Verification items for this drawing (mm, ordinates from the low corner). A direction names the side the tool comes from. Give positions to 0.01 mm unless a question says otherwise; leave off trailing zeros. Order: outer loops, then holes, each group sorted by start corner. A loop starts at its lowest first (then second) coordinate and runs counter-clockwise, first axis right, second up. Notation, with made-up numbers: (-7.5, -18) -> (7.5, -18) arc R19 ccw to (7.5, 19) -> close; hole circle Ø11 at (11.25, 9). An arc over 180 degrees is marked (long way). One line per question, with ' | ' between items.
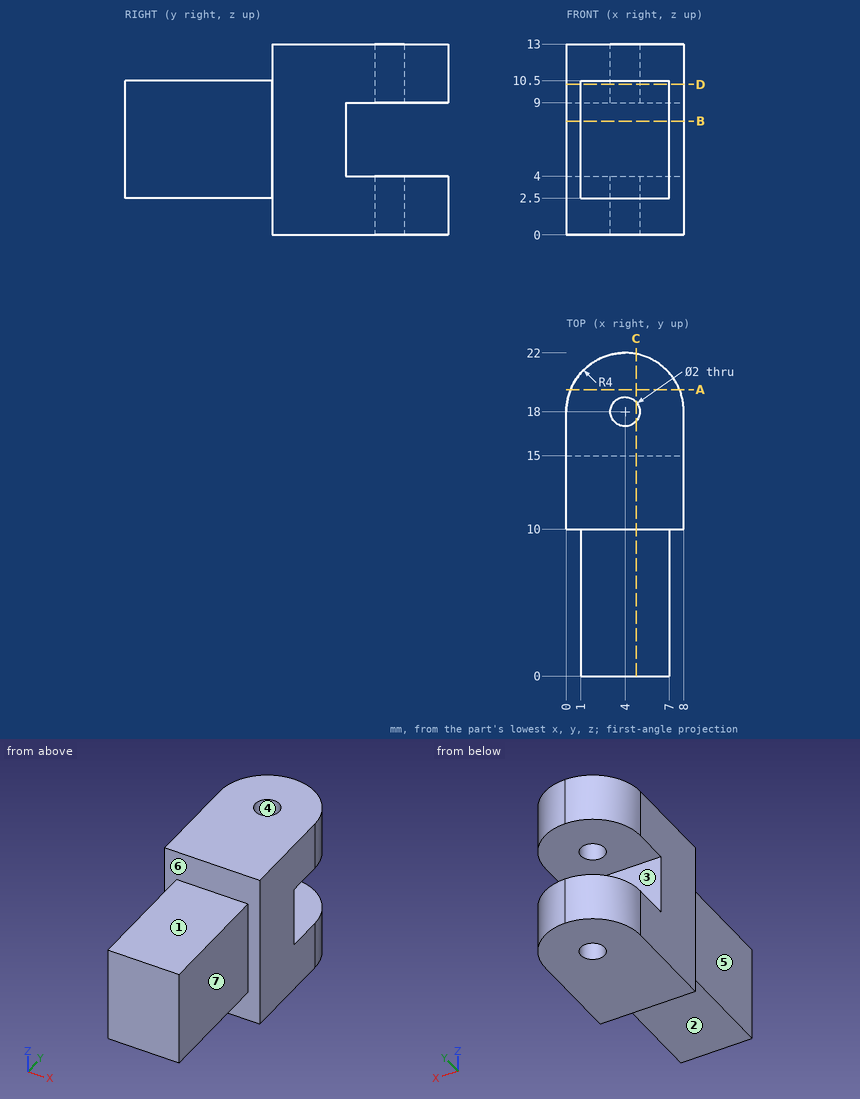
Q1. Section check B-B (z = 7.75). Enter the section's corners in (x, y), and give its area (3 significant figures).
Result sheet:
outline: (0, 10) -> (1, 10) -> (1, 0) -> (7, 0) -> (7, 10) -> (8, 10) -> (8, 15) -> (0, 15) -> close | area: 100 mm2
Q2. Access from +Z, -Z, +X, -X, +Y, -Y to the whole of each face (thin tool, end or side, straight path). Record for the marked faces 1, 2 and 3.
Result sheet:
face 1: +Z, +X, -X, -Y | face 2: -Z, +X, -X, -Y | face 3: +X, -X, +Y
Q3. Mould release check, pull along X, two halves, no side actions. Record for the marked faces 4, 5, 6 and 7: pulls with the +X half, pulls with the -X half, needs draft (parallel to the pull), parting line crosses it, or undercut.
Result sheet:
face 4: undercut | face 5: pulls with the -X half | face 6: needs draft | face 7: pulls with the +X half
Q4. Section check A-A (y = 19.5). Enter the section's corners in (x, z).
Result sheet:
outline: (0.29, 0) -> (7.71, 0) -> (7.71, 4) -> (0.29, 4) -> close; (0.29, 9) -> (7.71, 9) -> (7.71, 13) -> (0.29, 13) -> close
Q5. Section check D-D (z = 10.25). Enter the section's corners in (x, y).
Result sheet:
outline: (0, 10) -> (1, 10) -> (1, 0) -> (7, 0) -> (7, 10) -> (8, 10) -> (8, 18) arc R4 ccw to (0, 18) -> close; hole circle Ø2 at (4, 18)
Q6. Thickness scan on line 1 (Z direction, x = 3.5, y = 20); line 2 (Y direction, x = 4, z = 10.1); line 3 (Y direction, x = 4, z = 12.15). Record the ranges inside material, lowest first.
Result sheet:
line 1: z = 0 to 4, 9 to 13 | line 2: y = 0 to 17, 19 to 22 | line 3: y = 10 to 17, 19 to 22
Q7. Section check C-C (x = 4.75). Enter the section's corners in (y, z), and give its area (3 significant figures).
Result sheet:
outline: (0, 2.5) -> (10, 2.5) -> (10, 0) -> (17.34, 0) -> (17.34, 4) -> (15, 4) -> (15, 9) -> (17.34, 9) -> (17.34, 13) -> (10, 13) -> (10, 10.5) -> (0, 10.5) -> close; (18.66, 0) -> (21.93, 0) -> (21.93, 4) -> (18.66, 4) -> close; (18.66, 9) -> (21.93, 9) -> (21.93, 13) -> (18.66, 13) -> close | area: 190 mm2
Q8. Depth check by flat-ended pin: pin 1 Ø1 at (y, z) = (7.5, 10.5) entering from -X; pin 2 Ø1.8 at (x, y) = (3, 3) entering from -Z; pin 3 Ø4 at (y, z) = (6.5, 5.5) entering from +X; pin 4 Ø1.2 at (x, y) = (4, 18) entering from -Z. Enter the tip coordinate at first touch or a pass-through.
Result sheet:
pin 1: stops at x = 1 | pin 2: stops at z = 2.5 | pin 3: stops at x = 7 | pin 4: passes through
